Check sheet for the drawn part. Datum: minimum x, y, z corner. Units: mm. A direction names the side the tool comes from. Coordinates: 2 decimals unless noted, no trailing zeros. Loops run counter-clockwise (first coordinate to the right, second up) from the corner with the lowest first, then second, coordinate; pieces in that order, holes last.
Q1. Go/stop test with flat-tipped pins: P1, Ø1, axis at x = 17, z = 33.5, coming from the -Y side; P2, Ø6.5, axis at x = 10, z = 53, coming from the -Y side. Record where each tip stops, or that it passes through.
Q2. Sectioned sample at C-C (x = 19). Enter the section's corners in (y, z), then the cut area to 3 significant figures.
Q3. Sectioned sample at B-B (y = 2). Enter the section's corners in (x, z).
Q4. Access from +Z, -Z, +X, -X, +Y, -Y to the whole of each face (thin tool, end or side, straight path). Record for the marked faces 5 and 6.
Q5. Material ranges on probe 1 along Z at (x, y) = (8, 7); probe 2 along Z at (x, y) = (3, 1.5); probe 3 along Y at (x, z) = (3.25, 19.5), recorded low to high.
Q6. Sectioned sample at D-D (z = 16). Enter the section's corners in (x, y).
Q7. Sectioned sample at A-A (y = 12.25). Enter the section's corners in (x, z).
Q8. Mould release check, pull along Z, two halves, no side actions. Record for the marked faces 1, 2, 3 and 4: +Z half, -Z half, draft (parallel to the pull), parting line (faces both ways), or undercut.
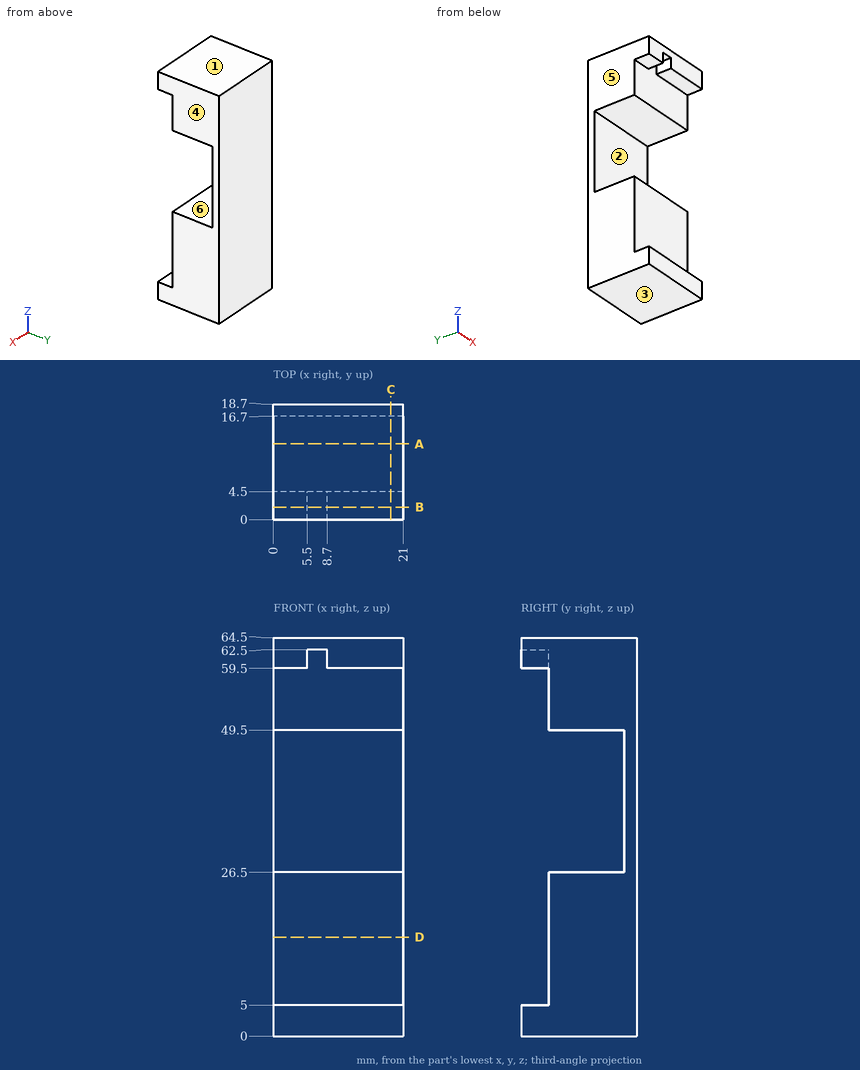
Geometry check:
1. P1: stops at y = 16.7
1. P2: stops at y = 4.5
2. outline: (0, 0) - (18.7, 0) - (18.7, 64.5) - (0, 64.5) - (0, 59.5) - (4.5, 59.5) - (4.5, 49.5) - (16.7, 49.5) - (16.7, 26.5) - (4.5, 26.5) - (4.5, 5) - (0, 5) - close
2. area: 680 mm2
3. outline: (0, 0) - (21, 0) - (21, 5) - (0, 5) - close; (0, 59.5) - (5.5, 59.5) - (5.5, 62.5) - (8.7, 62.5) - (8.7, 59.5) - (21, 59.5) - (21, 64.5) - (0, 64.5) - close
4. face 5: +Z, -Z, -X, +Y, -Y
4. face 6: +X, -X, -Y
5. probe 1: z = 0 to 26.5, 49.5 to 64.5
5. probe 2: z = 0 to 5, 59.5 to 64.5
5. probe 3: y = 4.5 to 18.7
6. outline: (0, 4.5) - (21, 4.5) - (21, 18.7) - (0, 18.7) - close
7. outline: (0, 0) - (21, 0) - (21, 26.5) - (0, 26.5) - close; (0, 49.5) - (21, 49.5) - (21, 64.5) - (0, 64.5) - close
8. face 1: +Z half
8. face 2: undercut
8. face 3: -Z half
8. face 4: draft
